Part model, mm, in its own coordinate system. Face numbers are marked on the shaded views. A direction names the side the tool comes from. Give positions to 0.01 mm unless a question says otherwise; leave off trailing zeros. Write each loop counter-clockwise with the first axis right and the second up, starting at its lowest first coordinate (ties: lowest second). Pieces come first, ordered by that corner, then holes.
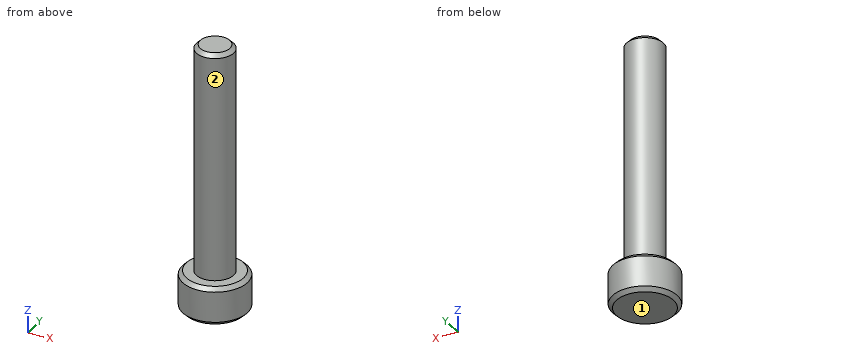
```python
from build123d import *

# Parameters (mm, degrees)
SKIZZE1_R                       = 4.25
SKIZZE1_R_2                     = 2.45
AUFSATZ_LINEAR_AUSTRAGEN1_DEPTH = 5
SKIZZE1_3_R                     = 2.45
AUFSATZ_LINEAR_AUSTRAGEN2_DEPTH = 35
FASE1_SIZE                      = 0.5


with BuildPart() as part:
    # Skizze1 → Aufsatz-Linear austragen1 (new body)
    # profile 1 of 2: a face of its own
    with BuildSketch(Plane.XY):
        Circle(SKIZZE1_R)
        Circle(SKIZZE1_R_2, mode=Mode.SUBTRACT)
    # profile 2 of 2: a face of its own
    with BuildSketch(Plane.XY):
        Circle(SKIZZE1_R_2)
    extrude(amount=AUFSATZ_LINEAR_AUSTRAGEN1_DEPTH)

    # Skizze1<3> → Aufsatz-Linear austragen2 (add)
    with BuildSketch(Plane.XY):
        Circle(SKIZZE1_3_R)
    extrude(amount=AUFSATZ_LINEAR_AUSTRAGEN2_DEPTH)

    # Fase1
    fase1_edges = [part.edges().sort_by_distance(p)[0] for p in [
        (-4.25, 0, 0),
        (-4.25, 0, 5),
        (-2.45, 0, 35),
    ]]
    chamfer(fase1_edges, length=FASE1_SIZE)


solid = part.part
```
1) Saw through at D-D, the plane z = 3. Write the cut outline in (x, y).
Answers follow:
outline: circle Ø8.5 at (0, 0)
2) Pin check, flat tip, straight feed: pin 1 Ø3 at (y, z) = (0, 24.5) entering from +X. Stop position of the tip, or through.
Answers follow:
pin 1: stops at x = 2.45
3) Saw through at A-A, the plane y = 0. Write the cut outline in (x, z), then the cut area to 3 significant figures.
Answers follow:
outline: (-4.25, 0.5) - (-3.75, 0) - (3.75, 0) - (4.25, 0.5) - (4.25, 4.5) - (3.75, 5) - (2.45, 5) - (2.45, 34.5) - (1.95, 35) - (-1.95, 35) - (-2.45, 34.5) - (-2.45, 5) - (-3.75, 5) - (-4.25, 4.5) - close
area: 189 mm2
4) Saw through at C-C, the plane z = 30.5. Write the cut outline in (x, y).
Answers follow:
outline: circle Ø4.9 at (0, 0)
5) Wall check: L1, parallel to Z at x = 2.75, y = 0.75; L2, parallel to Y at x = 0, z = 11.5; L3, parallel to X at y = 1.25, z = 7. Give the ranges that are in metal, low to high.
Answers follow:
L1: z = 0 to 5
L2: y = -2.45 to 2.45
L3: x = -2.11 to 2.11
6) 3-axis set-ups, long thin cutter, end or side, ignore diameter. For the marked faces 1 and 2: which of +Z, -Z, +X, -X, +Y, -Y reach the whole face in a straight line?
Answers follow:
face 1: -Z, +X, -X, +Y, -Y
face 2: +Z
